Geometry: see drawing. Coordinates: mm, zero at the bounding-box minimum. Round coordinates to 2 decimals unless told otherwise and drop trailing zeros. Loops run counter-clockwise (first coordinate to the right, second up) from the corner with the lowest first, then second, coordinate; pieces in that order, holes last. Notation, with made-up numbers: (56.5, 81.25) - (85.5, 81.25) arc R17 cw to (85.5, 113.25) - close; hole circle Ø1 at (17, -31.5). An arc over 180 degrees is marked (long way). Return JSON: item names as keys, results as strings. Group by question number.
1. Material intervals for probe 1 along Z at (x, y) = (5, 144); probe 2 along Y at (x, z) = (6, 46.5); probe 3 along Z at (x, y) = (3, 126), sorted ascending.
2. First-contact query: pin 1 Ø1.9 at (x, y) = (2.5, 147.5) entering from +Z; pin 2 Ø3 at (x, y) = (1.5, 146.5) entering from -Z; pin 3 Ø3 at (x, y) = (2, 6) entering from -Z. Flat tips, straight axial feed; report the tip coordinate or a pass-through.
3. Section A-A on x = 1.5. Return loops of the section in (y, z), and give its area (3 significant figures).
4. Section B-B on z = 52. Return loops of the section in (x, y), and give its area (3 significant figures).
5. Section C-C on y = 44. Return loops of the section in (x, z), and give its area (3 significant figures).
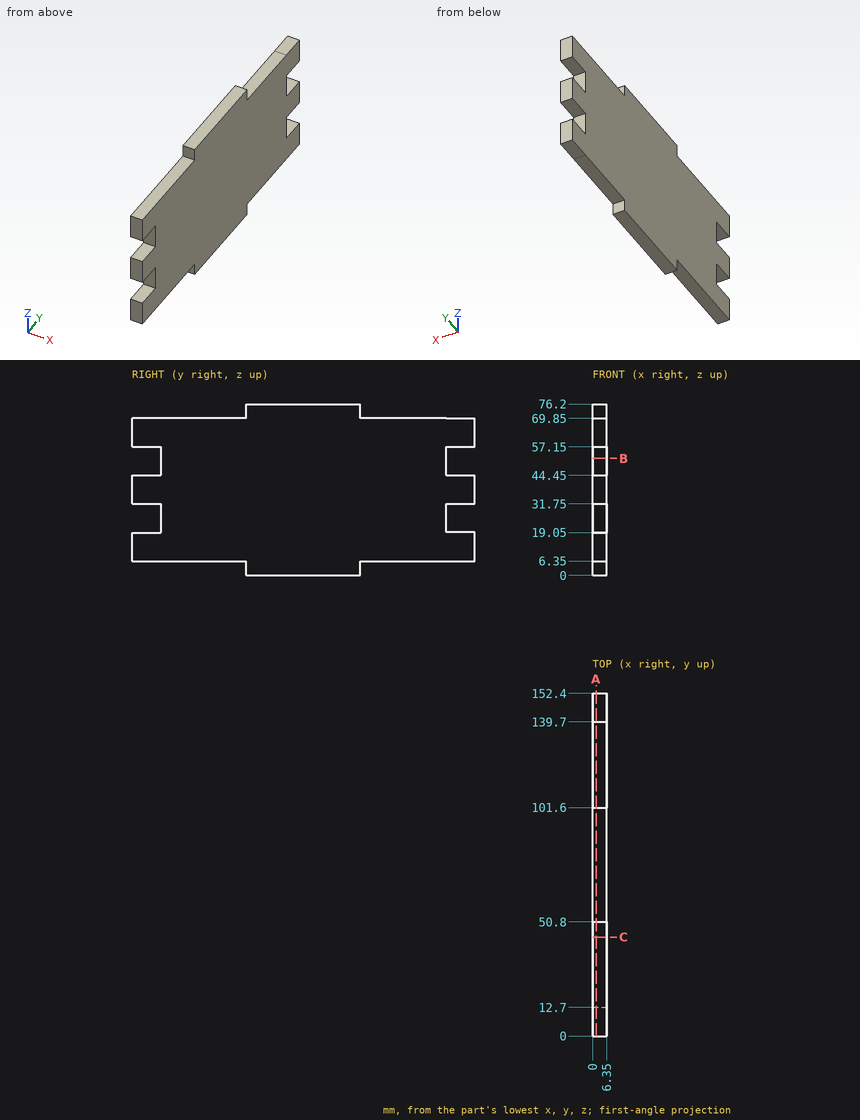
Taken from the geometry:
{
 "1": {"probe 1": "6.35 to 19.05, 31.75 to 44.45, 57.15 to 69.85", "probe 2": "12.7 to 139.7", "probe 3": "6.35 to 69.85"},
 "2": {"pin 1": "z = 69.85", "pin 2": "z = 6.35", "pin 3": "z = 6.35"},
 "3": {"outline": "(0, 6.35) - (50.8, 6.35) - (50.8, 0) - (101.6, 0) - (101.6, 6.35) - (152.4, 6.35) - (152.4, 19.05) - (139.7, 19.05) - (139.7, 31.75) - (152.4, 31.75) - (152.4, 44.45) - (139.7, 44.45) - (139.7, 57.15) - (152.4, 57.15) - (152.4, 69.85) - (101.6, 69.85) - (101.6, 76.2) - (50.8, 76.2) - (50.8, 69.85) - (0, 69.85) - (0, 57.15) - (12.7, 57.15) - (12.7, 44.45) - (0, 44.45) - (0, 31.75) - (12.7, 31.75) - (12.7, 19.05) - (0, 19.05) - close", "area": "9,680 mm2"},
 "4": {"outline": "(0, 12.7) - (6.35, 12.7) - (6.35, 139.7) - (0, 139.7) - close", "area": "806 mm2"},
 "5": {"outline": "(0, 6.35) - (6.35, 6.35) - (6.35, 69.85) - (0, 69.85) - close", "area": "403 mm2"}
}
